```python
from build123d import *

# Parameters (mm, degrees)
F1_DEPTH = 11.1125
F2_R     = 0.762
F3_R     = 2.54
F4_DEPTH = 14.479


with BuildPart() as f1:
    # F0 (on Top) → F1 (new body)
    with BuildSketch(Plane.XY):
        with BuildLine():
            Line((-6.35, -6.35), (-6.35, 0))
            ThreePointArc((-6.35, 0), (0, 6.35), (6.35, 0))
            Line((6.35, 0), (6.35, -6.35))
            Line((6.35, -6.35), (19.05, -6.35))
            Line((19.05, -6.35), (19.05, -4.572))
            Line((19.05, -4.572), (8.128, -4.572))
            Line((8.128, -4.572), (8.128, 0))
            ThreePointArc((8.128, 0), (0, 8.128), (-8.128, 0))
            Line((-8.128, 0), (-8.128, -4.572))
            Line((-8.128, -4.572), (-19.05, -4.572))
            Line((-19.05, -4.572), (-19.05, -6.35))
            Line((-19.05, -6.35), (-6.35, -6.35))
        make_face()
    extrude(amount=F1_DEPTH)

    # F2
    f2_edges = [f1.edges().sort_by_distance(p)[0] for p in [
        (-6.35, -6.35, 5.55625),
        (6.35, -6.35, 5.55625),
        (8.128, -4.572, 5.55625),
        (-8.128, -4.572, 5.55625),
    ]]
    fillet(f2_edges, radius=F2_R)

    # F3 (on face) → F4 (cut, through all)
    with BuildSketch(Plane.XZ.offset(6.35)):
        with Locations((-13.716, 5.55625)):
            Circle(F3_R)
        with Locations((13.716, 5.55625)):
            Circle(F3_R)
    extrude(amount=-F4_DEPTH, mode=Mode.SUBTRACT)


solid = f1.part
```
Part model, mm, in its own coordinate system. A direction names the side the tool comes from. Give positions to 0.01 mm unless a question says otherwise; leave off trailing zeros. Write each loop counter-clockwise with the first axis right and the second up, starting at its lowest first coordinate (ties: lowest second). Pieces come first, ordered by that corner, then holes. Notation, with made-up numbers: (-11, -12.75) -> (37, -12.75) arc R9 cw to (37, -4.75) -> close; hole circle Ø4 at (19, -16). An arc over 180 degrees is marked (long way). Put each result on its own line as item: value. Start each with the question number.
Item 1: Wall check: L1, parallel to X at y = -1.25, z = 3; L2, parallel to X at y = -5, z = 6.25; L3, parallel to Y at x = 10, z = 5.25. Give the ranges that are in metal, low to high. Write a range as [from, to].
Item 2: Cut at D-D (x = 0). List the corners of the cut face in (y, z), then the cut area to 3 significant figures.
Item 3: Cut at A-A (y = -1). List the corners of the cut face in (x, z), then the cut area to 3 significant figures.
Item 4: Pull direction Z, two halves, no side cores. Call faces 1 (the face through (-6, 3, 0)), 2 (the face through (10, -6.35, 5)), 3 (the face through (-16.254, -5.473, 5.668)): pulls with the +Z half, pulls with the -Z half, needs draft (parallel to the pull), parting line crosses it, or undercut.
Item 5: Cut at B-B (z = 9.25). List the corners of the cut face in (x, y).
Item 6: Cut at C-C (y = 5.5). List the corners of the cut face in (x, z), then the cut area to 3 significant figures.
Item 7: Which spindle directions (+Z, -Z, +X, -X, +Y, -Y) get a long thin tool onto all of the face, cutting with end or side? Do faces 4 (the face through (-8.128, -2, 5)), 5 (the face through (-6.35, -3, 5)), 6 (the face through (8.128, -2, 5)). Say none if no direction does.
Item 8: Pin check, flat tips, straight feed: pin 1 Ø1.1 at (y, z) = (-2.5, 7) entering from +X; pin 2 Ø5 at (x, z) = (11.5, 7.5) entering from +Y; pin 3 Ø5 at (y, z) = (-0.5, 9) entering from -X. Stop position of each tip, or through.
Answer list:
1. L1: x = [-8.13, -6.35], [6.35, 8.13]
1. L2: x = [-19.05, -16.16], [-11.27, -6.35], [6.35, 11.27], [16.16, 19.05]
1. L3: y = [-6.35, -4.57]
2. outline: (6.35, 0) -> (8.13, 0) -> (8.13, 11.11) -> (6.35, 11.11) -> close
2. area: 19.8 mm2
3. outline: (-8.13, 0) -> (-6.35, 0) -> (-6.35, 11.11) -> (-8.13, 11.11) -> close; (6.35, 0) -> (8.13, 0) -> (8.13, 11.11) -> (6.35, 11.11) -> close
3. area: 39.5 mm2
4. face 1: pulls with the -Z half
4. face 2: needs draft
4. face 3: undercut
5. outline: (-19.05, -6.35) -> (-7.11, -6.35) arc R0.76 ccw to (-6.35, -5.59) -> (-6.35, 0) arc R6.35 cw to (6.35, 0) -> (6.35, -5.59) arc R0.76 ccw to (7.11, -6.35) -> (19.05, -6.35) -> (19.05, -4.57) -> (8.89, -4.57) arc R0.76 cw to (8.13, -3.81) -> (8.13, 0) arc R8.13 ccw to (-8.13, 0) -> (-8.13, -3.81) arc R0.76 cw to (-8.89, -4.57) -> (-19.05, -4.57) -> close
6. outline: (-5.98, 0) -> (-3.17, 0) -> (-3.17, 11.11) -> (-5.98, 11.11) -> close; (3.17, 0) -> (5.98, 0) -> (5.98, 11.11) -> (3.17, 11.11) -> close
6. area: 62.5 mm2
7. face 4: +Z, -Z, -X, +Y
7. face 5: +Z, -Z, -Y
7. face 6: +Z, -Z, +X, +Y
8. pin 1: stops at x = 8.13
8. pin 2: stops at y = -4.57
8. pin 3: stops at x = -8.13
